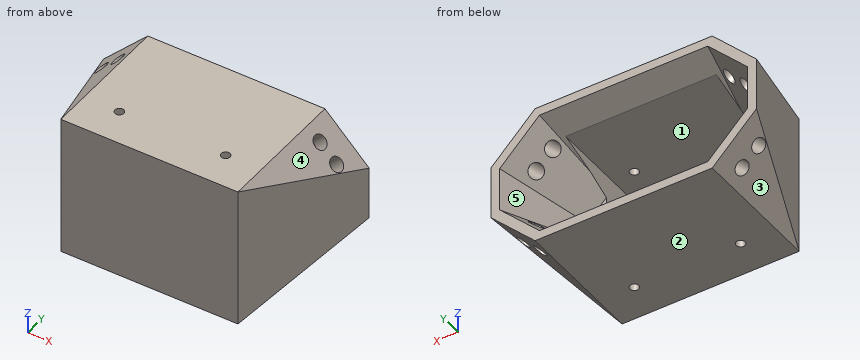
from build123d import *

# Parameters (mm, degrees)
BOSS_EXTRUDE1_DEPTH     = 150
CUT_EXTRUDE1_DEPTH      = 227.715680975
CUT_EXTRUDE1_DEPTH_BACK = 227.715680975
SKETCH3_W               = 170
SKETCH3_H               = 190
CUT_EXTRUDE2_DEPTH      = 60
CUT_EXTRUDE3_DEPTH      = 100
CUT_EXTRUDE3_DRAFT      = -18.43
SKETCH5_R               = 8.25
CUT_EXTRUDE4_DEPTH      = 80
MIRROR2_COPY_1_SKETCH_R = 8.25
MIRROR2_COPY_1_DEPTH    = 80
SKETCH7_R               = 5
CUT_EXTRUDE5_DEPTH      = 266.706605112


with BuildPart() as part:
    # Sketch1 → Boss-Extrude1 (new body)
    with BuildSketch(Plane(origin=(0, 0, 0), x_dir=(1, 0, 0), z_dir=(0, 1, 0))):
        Polygon((-150, 30), (-100, 80), (100, 80), (150, 30), (150, -30), (100, -80), (-100, -80), (-150, -30), align=None)
    extrude(amount=BOSS_EXTRUDE1_DEPTH)

    # Sketch2 → Cut-Extrude1 (cut, two sides: drawn at the far end of the back side and taken through both)
    with BuildSketch(Plane.XY.offset(-CUT_EXTRUDE1_DEPTH_BACK)):
        Polygon((-150, 150), (-100, 0), (-150, 0), align=None)
        Polygon((100, 0), (150, 150), (150, 0), align=None)
    extrude(amount=CUT_EXTRUDE1_DEPTH + CUT_EXTRUDE1_DEPTH_BACK, mode=Mode.SUBTRACT)

    # Sketch3 → Cut-Extrude2 (cut, symmetric)
    with BuildSketch(Plane.XY):
        with Locations((0, 105)):
            Rectangle(SKETCH3_W, SKETCH3_H)
    extrude(amount=CUT_EXTRUDE2_DEPTH, both=True, mode=Mode.SUBTRACT)


with BuildPart() as cut_extrude3_tool:
    # Sketch4 → Cut-Extrude3 (with draft: the straight prism first)
    with BuildSketch(Plane(origin=(0, 150, 0), x_dir=(1, 0, 0), z_dir=(0, 1, 0))):
        Polygon((-140, -25), (-125, -40), (-95, -70), (95, -70), (140, -25), (140, 25), (95, 70), (-95, 70), (-140, 25), align=None)
    extrude(amount=-CUT_EXTRUDE3_DEPTH)
    # Cut-Extrude3: the draft: its side faces are tilted about the plane it starts from
    cut_extrude3_sides = [cut_extrude3_tool.faces().sort_by_distance(p)[0] for p in [
        (-117.5, 100, 47.5),
        (-117.5, 100, -47.5),
        (0, 100, -70),
        (117.5, 100, -47.5),
        (140, 100, 0),
        (117.5, 100, 47.5),
        (0, 100, 70),
        (-140, 100, 0),
    ]]
    draft(cut_extrude3_sides, Plane(origin=(0, 150, 0), x_dir=(1, 0, 0), z_dir=(0, 1, 0)), CUT_EXTRUDE3_DRAFT)


with BuildPart() as part_1:
    add(part.part)

    # Cut-Extrude3: cut by cut_extrude3_tool
    add(cut_extrude3_tool.part, mode=Mode.SUBTRACT)

    # Sketch5 → Cut-Extrude4 (cut)
    with BuildSketch(Plane(origin=(-90, 0, 90), x_dir=(0.7071067811865475, 0, 0.7071067811865477), z_dir=(-0.7071067811865477, 0, 0.7071067811865475))):
        with Locations((-60.642135624, 120)):
            Circle(SKETCH5_R)
        with Locations((-34.142135624, 120)):
            Circle(SKETCH5_R)
    cut_extrude4 = extrude(amount=-CUT_EXTRUDE4_DEPTH, mode=Mode.SUBTRACT)

    # Mirror1: Cut-Extrude4 across plane
    add(cut_extrude4.mirror(Plane.XY), mode=Mode.SUBTRACT)

    # Mirror2: Cut-Extrude4 across plane
    add(cut_extrude4.mirror(Plane(origin=(0, 0, 0), x_dir=(0, 0, 1), z_dir=(1, 0, 0))), mode=Mode.SUBTRACT)

    # Mirror2 copy 1 sketch → Mirror2 copy 1 (cut)
    with BuildSketch(Plane(origin=(90, 0, -90), x_dir=(-0.7071067811865475, 0, -0.7071067811865477), z_dir=(0.7071067811865477, 0, -0.7071067811865475))):
        with Locations((-60.642135624, 120)):
            Circle(MIRROR2_COPY_1_SKETCH_R)
        with Locations((-34.142135624, 120)):
            Circle(MIRROR2_COPY_1_SKETCH_R)
    extrude(amount=-MIRROR2_COPY_1_DEPTH, mode=Mode.SUBTRACT)

    # Sketch7 → Cut-Extrude5 (cut, through all)
    with BuildSketch(Plane.XY.offset(80)):
        with Locations((-60, 40)):
            Circle(SKETCH7_R)
        with Locations((60, 40)):
            Circle(SKETCH7_R)
    extrude(amount=-CUT_EXTRUDE5_DEPTH, mode=Mode.SUBTRACT)


solid = part_1.part
Can you work these out from the model? Positions are in its coordinate system, mm. Face numbers are marked on the shaded views. A direction names the side the tool comes from. Coordinates: 2 decimals unless noted, no trailing zeros. Write each loop counter-clockwise with the first axis right and the second up, starting at its lowest first coordinate (ties: lowest second). Pieces come first, ordered by that corner, then holes. Notation, with made-up numbers: (28.5, 36) - (63.5, 36) arc R23 ccw to (63.5, 60) - close; hole circle Ø2 at (17, -23). An arc over 180 degrees is marked (long way). Return JSON: item names as keys, results as strings. Group by question number.
Item 1: I'm going to push flat-ended pins straight in: pin 1 Ø6 at (y, z) = (110.5, 0) entering from +X; pin 2 Ø12 at (y, z) = (98.5, -27.5) entering from +X; pin 3 Ø8 at (x, y) = (60, 40) entering from +Z; pin 4 Ø17.5 at (x, z) = (90.5, 4.5) entering from +Y. Where does each tip first touch, or does it pass through?
Item 2: If we section it at A-A (x = -60): Write out the boundary of the cut face in (y, z), then the cut area to 3 significant figures.
Item 3: We'd pull the mould along Z, two halves only. Please class the marked faces 3, 4 and 5: pulls with the +Z half, pulls with the -Z half, needs draft (parallel to the pull), parting line crosses it, or undercut.
Item 4: If we section it at C-C (z = -3): Write out the boundary of the cut face in (x, y).
Item 5: Which directions (+Z, -Z, +X, -X, +Y, -Y) give clear straight access to the entire face, cutting with the end or side of a thin tool? Please do the marked faces 1 and 2.
Item 6: If we section it at D-D (y = 40): Write out the boundary of the cut face in (x, z).
Item 7: If we section it at B-B (y = 138): Write out the boundary of the cut face in (x, z), then the cut area to 3 significant figures.
Item 8: Please list where these lines run through material, in increasing order: probe 1 along Y at (x, z) = (-60, 72.75); probe 2 along Z at (x, y) = (-35.5, 53.5); probe 3 along Y at (x, z) = (19.5, 22.5).
Return value:
{
 "1": {"pin 1": "stops at x = 137.83", "pin 2": "stops at x = 134.83", "pin 3": "passes through", "pin 4": "stops at y = 50"},
 "2": {"outline": "(0, -80) - (35, -80) - (35, -60) - (10, -60) - (10, 60) - (35, 60) - (35, 80) - (0, 80) - close; (45, -80) - (150, -80) - (150, -70) - (119.99, -60) - (45, -60) - close; (45, 60) - (119.99, 60) - (150, 70) - (150, 80) - (45, 80) - close", "area": "6,500 mm^2"},
 "3": {"face 3": "pulls with the -Z half", "face 4": "pulls with the +Z half", "face 5": "undercut"},
 "4": {"outline": "(-150, 150) - (-100, 0) - (100, 0) - (150, 150) - (140, 150) - (106.68, 50) - (85, 50) - (85, 10) - (-85, 10) - (-85, 50) - (-106.68, 50) - (-140, 150) - close"},
 "5": {"face 1": "+Y", "face 2": "-Z, +X, -X, +Y, -Y"},
 "6": {"outline": "(-113.33, -66.67) - (-100, -80) - (-65, -80) - (-65, -60) - (-85, -60) - (-85, 60) - (-65, 60) - (-65, 80) - (-100, 80) - (-113.33, 66.67) - close; (-55, -80) - (55, -80) - (55, -60) - (-55, -60) - close; (-55, 60) - (55, 60) - (55, 80) - (-55, 80) - close; (65, -80) - (100, -80) - (113.33, -66.67) - (113.33, 66.67) - (100, 80) - (65, 80) - (65, 60) - (85, 60) - (85, -60) - (65, -60) - close"},
 "7": {"outline": "(-146, -34) - (-100, -80) - (100, -80) - (146, -34) - (146, 34) - (100, 80) - (-100, 80) - (-146, 34) - close; hole (-136, -23.34) - (-93.34, -66) - (93.34, -66) - (136, -23.34) - (136, 23.34) - (93.34, 66) - (-93.34, 66) - (-136, 23.34) - close", "area": "10,200 mm^2"},
 "8": {"probe 1": "y = 0 to 35, 45 to 150", "probe 2": "z = -80 to -60, 60 to 80", "probe 3": "y = 0 to 10"}
}
